CAD build for the part. Positions are in the model's coordinates, mm. Round coordinates to 2 decimals unless told otherwise and drop trailing zeros. Write each loop counter-clockwise with the first axis right and the second up, starting at its lowest first coordinate (ties: lowest second). Pieces come first, ordered by that corner, then holes. Notation, with made-up numbers: (-32, 32.5) - (22, 32.5) arc R23 ccw to (22, 58.5) - close; hole circle Ø10 at (-10.75, -11.5). An arc over 180 degrees is marked (long way). Put each result on its own line as item: value. Start each with the question number.
Item 1: Cut at D-D (y = 4.25). Give the cut face in (x, z).
Item 2: Pin check, flat tips, straight feed: pin 1 Ø3 at (x, z) = (2, 18) entering from -Y; pin 2 Ø1 at (x, z) = (3, 8) entering from +Y. Stop position of each tip, or through.
Item 3: Cut at C-C (z = 11.75). Give the cut face in (x, y), and give its area (3 significant figures).
Item 4: Drill centre lines: line 1 (Y direction, x = 0, z = 19.6); line 2 (Y direction, x = -1.25, z = 19); line 3 (X direction, y = 2.25, z = 2). Where is each one in solid material? Low to high. Write a range as from..to.
Item 5: Cut at A-A (x = 0). Give the cut face in (y, z), and give its area (3 significant figures).
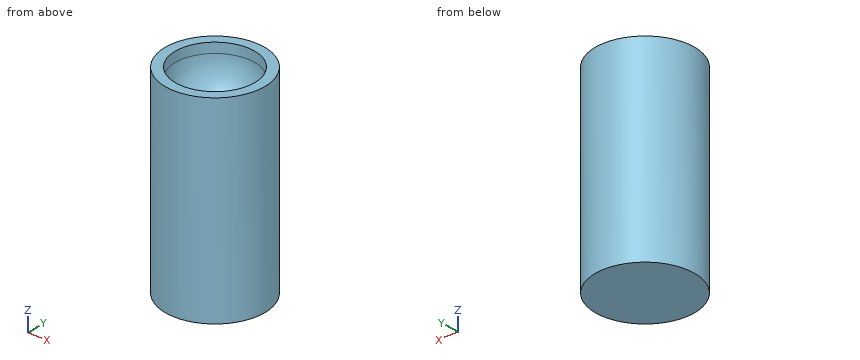
```python
from build123d import *

# Parameters (mm, degrees)
SCHIZZO1_R                   = 5
ESTRUSIONE_ESTRUSIONE1_DEPTH = 20
SCHIZZO2_R                   = 4
TAGLIO_ESTRUSIONE1_DEPTH     = 1


with BuildPart() as part:
    # Schizzo1 → Estrusione-Estrusione1 (new body)
    with BuildSketch(Plane.XY):
        Circle(SCHIZZO1_R)
    extrude(amount=ESTRUSIONE_ESTRUSIONE1_DEPTH)

    # Schizzo2 → Taglio-Estrusione1 (cut)
    with BuildSketch(Plane.XY.offset(20)):
        Circle(SCHIZZO2_R)
    extrude(amount=-TAGLIO_ESTRUSIONE1_DEPTH, mode=Mode.SUBTRACT)

    # Schizzo15 → Taglia-Rivoluzione2 (revolve, cut)
    with BuildSketch(Plane.XY.offset(19)):
        with BuildLine():
            Line((0, -4), (0, 4))
            ThreePointArc((0, 4), (-4, 0), (0, -4))
        make_face()
    revolve(axis=Axis((0, -4, 19), (0, 1, 0)), mode=Mode.SUBTRACT)


solid = part.part
```
Output values:
1. outline: (-2.63, 0) - (2.63, 0) - (2.63, 20) - (-2.63, 20) - close
2. pin 1: y = -4.97
2. pin 2: y = 4.33
3. outline: circle Ø10 at (0, 0)
3. area: 78.5 mm2
4. line 1: -5..-4, 4..5
4. line 2: -4.84..-3.8, 3.8..4.84
4. line 3: -4.47..4.47
5. outline: (-5, 0) - (5, 0) - (5, 20) - (4, 20) - (4, 19) arc R4 cw to (-4, 19) - (-4, 20) - (-5, 20) - close
5. area: 167 mm2
